```python
from build123d import *

# Parameters (mm, degrees)
SKETCH_W        = 65
SKETCH_H        = 56.5
SKETCH_W_2      = 63
SKETCH_H_2      = 54.5
PAD_DEPTH       = 25
SKETCH001_W     = 52
SKETCH001_H     = 1
POCKET_DEPTH    = 10
SKETCH002_W     = 14
SKETCH002_H     = 1
POCKET001_DEPTH = 6
SKETCH003_W     = 6.25
SKETCH003_H     = 6.25
PAD001_DEPTH    = 25
SKETCH004_R     = 1
POCKET002_DEPTH = 10


with BuildPart() as part:
    # Sketch → Pad (new body)
    with BuildSketch(Plane.XZ):
        with Locations((32.5, -28.25)):
            Rectangle(SKETCH_W, SKETCH_H)
        with Locations((32.5, -28.25)):
            Rectangle(SKETCH_W_2, SKETCH_H_2, mode=Mode.SUBTRACT)
    extrude(amount=PAD_DEPTH)

    # Sketch001 → Pocket (cut)
    with BuildSketch(Plane.XZ):
        with Locations((32.5, -0.5)):
            Rectangle(SKETCH001_W, SKETCH001_H)
    extrude(amount=POCKET_DEPTH, mode=Mode.SUBTRACT)

    # Sketch002 → Pocket001 (cut)
    with BuildSketch(Plane.XZ):
        with Locations((51, -56)):
            Rectangle(SKETCH002_W, SKETCH002_H)
    extrude(amount=POCKET001_DEPTH, mode=Mode.SUBTRACT)

    # Sketch003 → Pad001 (join)
    with BuildSketch(Plane.XZ):
        with Locations((3.125, -3.125)):
            Rectangle(SKETCH003_W, SKETCH003_H)
        with Locations((3.125, -53.375)):
            Rectangle(SKETCH003_W, SKETCH003_H)
        with Locations((61.875, -53.375)):
            Rectangle(SKETCH003_W, SKETCH003_H)
        with Locations((61.875, -3.125)):
            Rectangle(SKETCH003_W, SKETCH003_H)
    extrude(amount=PAD001_DEPTH)

    # Sketch004 → Pocket002 (cut)
    with BuildSketch(Plane.XZ):
        with Locations((4.5, -52)):
            Circle(SKETCH004_R)
        with Locations((4.5, -4.5)):
            Circle(SKETCH004_R)
        with Locations((60.5, -4.5)):
            Circle(SKETCH004_R)
        with Locations((60.5, -52)):
            Circle(SKETCH004_R)
    extrude(amount=POCKET002_DEPTH, mode=Mode.SUBTRACT)


solid = part.part
```
Check sheet for the modelled part. Datum: model origin and axes. Units: mm. A direction names the side the tool comes from. Round coordinates to 2 decimals unless told otherwise and drop trailing zeros. Loops run counter-clockwise (first coordinate to the right, second up) from the corner with the lowest first, then second, coordinate; pieces in that order, holes last. Notation, with made-up numbers: (-10.5, 60.25) - (7.5, 60.25) arc R21 cw to (7.5, 98.25) - close; hole circle Ø11 at (66, 17). An arc over 180 degrees is marked (long way). Answer as a JSON object with one key per item and string values. Group by question number.
Q1. Scan lines: line 1 along Z through (x, y) = (60.5, -6.5); line 2 along X through (y, z) = (-13, -36.5); line 3 along X through (y, z) = (-12.5, -4). Record each from-to range of solid material in increasing order. Write a range as [from, to].
Q2. Sectioned sample at C-C, the plane x = 4.5. Enter the section's corners in (y, z), plus the area to 4 significant figures.
Q3. Gauge pin test, flat ends, axial feed: P1, Ø10, axis at x = 52.5, z = -10, coming from the +Y side; P2, Ø0.5, axis at x = 28.5, z = -0.5, coming from the +Y side. Record the tip position at first contact, or that the pin passes through.
Q4. Sectioned sample at A-A, the plane y = -2.25. Enter the section's corners in (x, z), plus the area to 3 significant figures.
Q5. Mould release check, pull along X, two halves, no side actions. Record for faces 4 (the face through (61, -12, -50.25)), 5 (the face through (65, -12, -29)), 6 (the face through (64.3, 0, -28.1)): released by +X, released by -X, zero draft, split by the parting line, or undercut.
Q6. Sectioned sample at B-B, the plane z = -10.5. Enter the section's corners in (x, y), plus the area to 3 significant figures.
Q7. Set-up check for faces 1 (the face through (61, -12, -6.25)), 2 (the face through (32, -12, -56.5)), 3 (the face through (4.37, -4.93, -51.01)): record each of +Z, -Z, +X, -X, +Y, -Y from which the full face is reachable in a straight line by a thin tool's end or side.
Q8. Sectioned sample at D-D, the plane y = -18.25. Enter the section's corners in (x, z), plus the area to 3 significant figures.
Solution:
{
 "1": {"line 1": "z = [-56.5, -53], [-51, -50.25], [-6.25, -5.5], [-3.5, 0]", "line 2": "x = [0, 1], [64, 65]", "line 3": "x = [0, 6.25], [58.75, 65]"},
 "2": {"outline": "(-25, -56.5) - (0, -56.5) - (0, -53) - (-10, -53) - (-10, -51) - (0, -51) - (0, -50.25) - (-25, -50.25) - close; (-25, -6.25) - (0, -6.25) - (0, -5.5) - (-10, -5.5) - (-10, -3.5) - (0, -3.5) - (0, 0) - (-25, 0) - close", "area": "272.5 mm²"},
 "3": {"P1": "passes through", "P2": "stops at y = -10"},
 "4": {"outline": "(0, -56.5) - (44, -56.5) - (44, -55.5) - (6.25, -55.5) - (6.25, -50.25) - (1, -50.25) - (1, -6.25) - (6.25, -6.25) - (6.25, -1) - (6.5, -1) - (6.5, 0) - (0, 0) - close; (58, -56.5) - (65, -56.5) - (65, 0) - (58.5, 0) - (58.5, -1) - (58.75, -1) - (58.75, -6.25) - (64, -6.25) - (64, -50.25) - (58.75, -50.25) - (58.75, -55.5) - (58, -55.5) - close; hole circle Ø2 at (4.5, -52); hole circle Ø2 at (4.5, -4.5); hole circle Ø2 at (60.5, -52); hole circle Ø2 at (60.5, -4.5)", "area": "271 mm²"},
 "5": {"face 4": "undercut", "face 5": "released by +X", "face 6": "zero draft"},
 "6": {"outline": "(0, -25) - (1, -25) - (1, 0) - (0, 0) - close; (64, -25) - (65, -25) - (65, 0) - (64, 0) - close", "area": "50.0 mm²"},
 "7": {"face 1": "+Y, -Y", "face 2": "-Z, +X, -X, +Y, -Y", "face 3": "+Y"},
 "8": {"outline": "(0, -56.5) - (65, -56.5) - (65, 0) - (0, 0) - close; hole (1, -50.25) - (6.25, -50.25) - (6.25, -55.5) - (58.75, -55.5) - (58.75, -50.25) - (64, -50.25) - (64, -6.25) - (58.75, -6.25) - (58.75, -1) - (6.25, -1) - (6.25, -6.25) - (1, -6.25) - close", "area": "349 mm²"}
}
